from build123d import *

# Parameters (mm, degrees)
F1_DEPTH     = 10.16
F2_C1_SIZE2  = 10.16
F2_C1_SIZE   = 9.4743532752
F2_C2_SIZE2  = 10.16
F2_C2_SIZE   = 9.4743532752
F2_C3_SIZE2  = 10.16
F2_C3_SIZE   = 9.4743532752
F2_C4_SIZE2  = 9.4743532752
F2_C4_SIZE   = 10.16
F2_C5_SIZE2  = 10.16
F2_C5_SIZE   = 9.4743532752
F2_C6_SIZE2  = 9.4743532752
F2_C6_SIZE   = 10.16
F2_C7_SIZE2  = 10.16
F2_C7_SIZE   = 9.4743532752
F2_C8_SIZE2  = 9.4743532752
F2_C8_SIZE   = 10.16
F2_C9_SIZE2  = 10.16
F2_C9_SIZE   = 9.4743532752
F2_C10_SIZE2 = 9.4743532752
F2_C10_SIZE  = 10.16
F2_C11_SIZE2 = 9.4743532752
F2_C11_SIZE  = 10.16
F2_C12_SIZE2 = 10.16
F2_C12_SIZE  = 9.4743532752


with BuildPart() as f1:
    # F0 (on Top) → F1 (new body, symmetric)
    with BuildSketch(Plane.XY):
        Polygon((-24.2152860866, 16.5479078158), (-26.4385515912, -12.697099003), (-2.2232655046, -29.2450068188), (24.2152860866, -16.5479078158), (26.4385515912, 12.697099003), (2.2232655046, 29.2450068188), align=None)
    extrude(amount=F1_DEPTH, both=True)

    # F2: chamfer of 10.16 x 9.4743532752 on 12 edges, made by hand

    # F2_c1
    f2_c1_edges = [f1.edges().sort_by_distance(p)[0] for p in [
        (-25.3269188389, 1.9254044064, -10.16),
    ]]
    f2_c1_side = f1.faces().sort_by_distance((-25.3269188389, 1.9254044064, -9.9705129345))[0]
    chamfer(f2_c1_edges, length=F2_C1_SIZE, length2=F2_C1_SIZE2, reference=f2_c1_side)

    # F2_c2
    f2_c2_edges = [f1.edges().sort_by_distance(p)[0] for p in [
        (-25.3269188389, 1.9254044064, 10.16),
    ]]
    f2_c2_side = f1.faces().sort_by_distance((-25.3269188389, 1.9254044064, 9.9705129345))[0]
    chamfer(f2_c2_edges, length=F2_C2_SIZE, length2=F2_C2_SIZE2, reference=f2_c2_side)

    # F2_c3
    f2_c3_edges = [f1.edges().sort_by_distance(p)[0] for p in [
        (-5.7082999727, 25.4358771179, -10.16),
    ]]
    f2_c3_side = f1.faces().sort_by_distance((-5.7082999727, 25.4358771179, -9.9705129345))[0]
    chamfer(f2_c3_edges, length=F2_C3_SIZE, length2=F2_C3_SIZE2, reference=f2_c3_side)

    # F2_c4
    f2_c4_edges = [f1.edges().sort_by_distance(p)[0] for p in [
        (-5.7082999727, 25.4358771179, 10.16),
    ]]
    f2_c4_side = f1.faces().sort_by_distance((-5.7082999727, 25.4358771179, 9.9705129345))[0]
    chamfer(f2_c4_edges, length=F2_C4_SIZE, length2=F2_C4_SIZE2, reference=f2_c4_side)

    # F2_c5
    f2_c5_edges = [f1.edges().sort_by_distance(p)[0] for p in [
        (19.1739657652, 17.6614713477, -10.16),
    ]]
    f2_c5_side = f1.faces().sort_by_distance((19.1739657652, 17.6614713477, -9.9705129345))[0]
    chamfer(f2_c5_edges, length=F2_C5_SIZE, length2=F2_C5_SIZE2, reference=f2_c5_side)

    # F2_c6
    f2_c6_edges = [f1.edges().sort_by_distance(p)[0] for p in [
        (18.8471324661, 17.8848181744, 10.16),
    ]]
    f2_c6_side = f1.faces().sort_by_distance((18.8471324661, 17.8848181744, 9.9705129345))[0]
    chamfer(f2_c6_edges, length=F2_C6_SIZE, length2=F2_C6_SIZE2, reference=f2_c6_side)

    # F2_c7
    f2_c7_edges = [f1.edges().sort_by_distance(p)[0] for p in [
        (24.882265738, -7.7744057701, -10.16),
    ]]
    f2_c7_side = f1.faces().sort_by_distance((24.882265738, -7.7744057701, -9.9705129345))[0]
    chamfer(f2_c7_edges, length=F2_C7_SIZE, length2=F2_C7_SIZE2, reference=f2_c7_side)

    # F2_c8
    f2_c8_edges = [f1.edges().sort_by_distance(p)[0] for p in [
        (24.9122731142, -7.3796864169, 10.16),
    ]]
    f2_c8_side = f1.faces().sort_by_distance((24.9122731142, -7.3796864169, 9.9705129345))[0]
    chamfer(f2_c8_edges, length=F2_C8_SIZE, length2=F2_C8_SIZE2, reference=f2_c8_side)

    # F2_c9
    f2_c9_edges = [f1.edges().sort_by_distance(p)[0] for p in [
        (5.7082999727, -25.4358771179, -10.16),
    ]]
    f2_c9_side = f1.faces().sort_by_distance((5.7082999727, -25.4358771179, -9.9705129345))[0]
    chamfer(f2_c9_edges, length=F2_C9_SIZE, length2=F2_C9_SIZE2, reference=f2_c9_side)

    # F2_c10
    f2_c10_edges = [f1.edges().sort_by_distance(p)[0] for p in [
        (6.0651406481, -25.2645045914, 10.16),
    ]]
    f2_c10_side = f1.faces().sort_by_distance((6.0651406481, -25.2645045914, 9.9705129345))[0]
    chamfer(f2_c10_edges, length=F2_C10_SIZE, length2=F2_C10_SIZE2, reference=f2_c10_side)

    # F2_c11
    f2_c11_edges = [f1.edges().sort_by_distance(p)[0] for p in [
        (-14.0040752488, -21.1943997376, 10.16),
    ]]
    f2_c11_side = f1.faces().sort_by_distance((-14.0040752488, -21.1943997376, 9.9705129345))[0]
    chamfer(f2_c11_edges, length=F2_C11_SIZE, length2=F2_C11_SIZE2, reference=f2_c11_side)

    # F2_c12
    f2_c12_edges = [f1.edges().sort_by_distance(p)[0] for p in [
        (-14.3309085479, -20.9710529109, -10.16),
    ]]
    f2_c12_side = f1.faces().sort_by_distance((-14.3309085479, -20.9710529109, -9.9705129345))[0]
    chamfer(f2_c12_edges, length=F2_C12_SIZE, length2=F2_C12_SIZE2, reference=f2_c12_side)


solid = f1.part
Input: part model. Units: mm. Frame: model coordinates. Coordinates: 2 decimals unless noted, no trailing zeros. Loops run counter-clockwise (first coordinate to the right, second up) from the corner with the lowest first, then second, coordinate; pieces in that order, holes last.
Q1. Material intervals for line 1 (Z direction, x = 13.5, y = -13.5); line 2 (Y direction, x = -2, z = 7); line 3 (X direction, y = 14, z = -6.5), sorted ascending.
Q2. Cut plane B-B (x = -4.5). Output: boundary loops of the cut face in (y, z), then the cut area to 3 significant figures.
Q3. Cut plane C-C (z = -2). Output: boundary loops of the cut face in (x, y).
Q4. Contact query for flat-ended pins moving along their axis: pin 1 (6 mm diameter, centred on x = 18.5, z = -3.5, fed in from -Y); pin 2 (8 mm diameter, centred on x = 2, z = 6.5, fed in from +Y); pin 3 (1.5 mm diameter, centred on y = 9, z = 5.5, fed in from -X). Output: stop coordinate, or through.
Q5. Cut plane A-A (y = -6.5). Output: boundary loops of the cut face in (x, z), then the cut area to 3 significant figures.
Q6. Cut plane D-D (y = 21). Output: boundary loops of the cut face in (x, z), then the cut area to 3 significant figures.
Working result:
1. line 1: z = -7.57 to 7.92
1. line 2: y = -21.49 to 19.98
1. line 3: x = -15.12 to 13.48
2. outline: (-27.69, -0.69) - (-15.38, -10.16) - (14.75, -10.16) - (26.02, -0.69) - (26.02, 0) - (15.51, 10.16) - (-16.21, 10.16) - (-27.69, 0) - close
2. area: 868 mm2
3. outline: (-24.97, -11.99) - (-2.1, -27.62) - (22.87, -15.63) - (24.97, 11.99) - (2.1, 27.62) - (-22.87, 15.63) - close
4. pin 1: stops at y = -19.79
4. pin 2: stops at y = 26.56
4. pin 3: stops at x = -20.42
5. outline: (-25.97, -0.69) - (-15.78, -10.16) - (14.79, -10.16) - (24.98, -0.69) - (24.98, 0) - (15.48, 10.16) - (-15.78, 10.16) - (-25.97, 0.69) - close
5. area: 842 mm2
6. outline: (-14.94, -0.69) - (1.6, -7.36) - (14.29, -0.69) - (14.29, 0) - (1.6, 7.68) - (-14.94, 0) - close
6. area: 230 mm2
